from build123d import *

# Parameters (mm, degrees)
BOSS_EXTRUDE7_DEPTH = 3.6
SKETCH3_R           = 11.2
SKETCH3_R_2         = 5.25
BOSS_EXTRUDE8_DEPTH = 2
SKETCH4_R           = 2
CUT_EXTRUDE1_DEPTH  = 31.753353097
FILLET5_R           = 30
SKETCH5_R           = 1.8
BOSS_EXTRUDE9_DEPTH = 3.6
SKETCH6_R           = 2
CUT_EXTRUDE3_DEPTH  = 10


with BuildPart() as part:
    # Sketch1 → Boss-Extrude7 (new body)
    with BuildSketch(Plane(origin=(0, 0, 0), x_dir=(1, 0, 0), z_dir=(0, 1, 0))):
        with BuildLine():
            ThreePointArc((4.41085686, -11.428335039), (-4.687872046, -11.317524273), (-11.2, -4.962106408))
            Line((-11.2, -4.962106408), (-11.2, -17.382337649))
            ThreePointArc((-11.2, -17.382337649), (-8.730733729, -21.077855779), (-4.371572875, -20.210764774))
            Line((-4.371572875, -20.210764774), (4.41085686, -11.428335039))
        make_face()
        with BuildLine():
            ThreePointArc((7.91959592, -7.919595979), (-4.286054462, -10.347450756), (-11.2, 0))
            Line((-11.2, 0), (-11.2, -4.962106408))
            ThreePointArc((-11.2, -4.962106408), (-4.687872046, -11.317524273), (4.41085686, -11.428335039))
            Line((4.41085686, -11.428335039), (7.91959592, -7.919595979))
        make_face()
        with BuildLine():
            Line((11.428335039, -4.41085686), (7.91959592, -7.919595979))
            Line((7.91959592, -7.919595979), (4.41085686, -11.428335039))
            ThreePointArc((4.41085686, -11.428335039), (8.66205807, -8.66205807), (11.428335039, -4.41085686))
        make_face()
        with BuildLine():
            Line((4.962106408, 11.2), (0, 11.2))
            ThreePointArc((0, 11.2), (7.919595949, 7.919595949), (11.2, 0))
            ThreePointArc((11.2, 0), (10.347450756, -4.286054462), (7.91959592, -7.919595979))
            Line((7.91959592, -7.919595979), (11.428335039, -4.41085686))
            ThreePointArc((11.428335039, -4.41085686), (12.042831981, -2.243367532), (12.25, 0))
            ThreePointArc((12.25, 0), (10.267626393, 6.681193625), (4.962106408, 11.2))
        make_face()
        with BuildLine():
            Line((17.382337649, 11.2), (4.962106408, 11.2))
            ThreePointArc((4.962106408, 11.2), (10.267626393, 6.681193625), (12.25, 0))
            ThreePointArc((12.25, 0), (12.042831981, -2.243367532), (11.428335039, -4.41085686))
            Line((11.428335039, -4.41085686), (20.210764774, 4.371572875))
            ThreePointArc((20.210764774, 4.371572875), (21.077855779, 8.730733729), (17.382337649, 11.2))
        make_face()
        with BuildLine():
            ThreePointArc((-11.2, 0), (-7.919595949, 7.919595949), (0, 11.2))
            Line((0, 11.2), (4.962106408, 11.2))
            ThreePointArc((4.962106408, 11.2), (-8.66205807, 8.66205807), (-11.2, -4.962106408))
            Line((-11.2, -4.962106408), (-11.2, 0))
        make_face()
    extrude(amount=BOSS_EXTRUDE7_DEPTH)

    # Sketch3 → Boss-Extrude8 (add)
    # profile 1 of 2: a face of its own
    with BuildSketch(Plane(origin=(0, 3.6, 0), x_dir=(1, 0, 0), z_dir=(0, 1, 0))):
        with BuildLine():
            Line((-4.371572875, -20.210764774), (4.41085686, -11.428335039))
            ThreePointArc((4.41085686, -11.428335039), (8.66205807, -8.66205807), (11.428335039, -4.41085686))
            Line((11.428335039, -4.41085686), (20.210764774, 4.371572875))
            ThreePointArc((20.210764774, 4.371572875), (21.077855779, 8.730733729), (17.382337649, 11.2))
            Line((17.382337649, 11.2), (4.962106408, 11.2))
            ThreePointArc((4.962106408, 11.2), (-8.66205807, 8.66205807), (-11.2, -4.962106408))
            Line((-11.2, -4.962106408), (-11.2, -17.382337649))
            ThreePointArc((-11.2, -17.382337649), (-8.730733729, -21.077855779), (-4.371572875, -20.210764774))
        make_face()
        with Locations(Location((0, 0, 0), (0, 0, 270))):
            Circle(SKETCH3_R, mode=Mode.SUBTRACT)
    # profile 2 of 2: a face of its own
    with BuildSketch(Plane(origin=(0, 3.6, 0), x_dir=(1, 0, 0), z_dir=(0, 1, 0))):
        with Locations(Location((0, 0, 0), (0, 0, 270))):
            Circle(SKETCH3_R)
        with Locations(Location((0, 0, 0), (0, 0, 270))):
            Circle(SKETCH3_R_2, mode=Mode.SUBTRACT)
    extrude(amount=BOSS_EXTRUDE8_DEPTH)

    # Sketch4 → Cut-Extrude1 (cut, through all)
    with BuildSketch(Plane(origin=(0, 0, 0), x_dir=(1, 0, 0), z_dir=(0, 1, 0))):
        with Locations(Location((-7.2, -17.382337649, 0), (0, 0, 270))):
            Circle(SKETCH4_R)
        with Locations(Location((17.382337649, 7.2, 0), (0, 0, 270))):
            Circle(SKETCH4_R)
    extrude(amount=CUT_EXTRUDE1_DEPTH, mode=Mode.SUBTRACT)

    # Fillet5
    fillet5_edges = [part.edges().sort_by_distance(p)[0] for p in [
        (4.41085686, 2.8, 11.428335039),
        (-11.2, 2.8, 4.962106408),
        (4.962106408, 2.8, -11.2),
        (11.428335039, 2.8, 4.41085686),
    ]]
    fillet(fillet5_edges, radius=FILLET5_R)

    # Sketch5 → Boss-Extrude9 (add)
    with BuildSketch(Plane.XZ.offset(-3.6)):
        with Locations(Location((-8.1, 0, 0), (0, 0, 90))):
            Circle(SKETCH5_R)
        with Locations(Location((8.1, 0, 0), (0, 0, 90))):
            Circle(SKETCH5_R)
        with Locations(Location((0, -8.1, 0), (0, 0, 90))):
            Circle(SKETCH5_R)
        with Locations(Location((0, 8.1, 0), (0, 0, 90))):
            Circle(SKETCH5_R)
    extrude(amount=BOSS_EXTRUDE9_DEPTH)

    # Sketch6 → Cut-Extrude3 (cut)
    with BuildSketch(Plane.XZ):
        with Locations(Location((0, 8.1, 0), (0, 0, 90))):
            Circle(SKETCH6_R)
    cut_extrude3 = extrude(amount=-CUT_EXTRUDE3_DEPTH, mode=Mode.SUBTRACT)

    # Mirror1: Cut-Extrude3 across plane
    add(cut_extrude3.mirror(Plane(origin=(0, 0, 0), x_dir=(0.707106781186546, 0, 0.707106781186549), z_dir=(-0.707106781186549, 0, 0.707106781186546))), mode=Mode.SUBTRACT)


solid = part.part
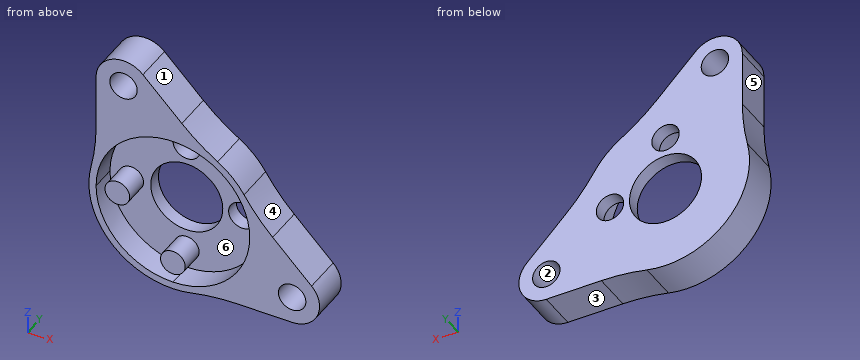
Model file for the job. Use its own axes, mm. Face numbers are marked on the shaded views. A direction names the side the tool comes from. Give positions to 0.01 mm unless a question says otherwise; leave off trailing zeros. Loops run counter-clockwise (first coordinate to the right, second up) from the corner with the lowest first, then second, coordinate; pieces in that order, holes last. Notation, with made-up numbers: (-32.75, 65) -> (-6.75, 65) arc R21 cw to (-6.75, 92) -> close; hole circle Ø3 at (19, 83.5). An arc over 180 degrees is marked (long way). Use a Markdown table: item, result. Add a question column.
(1) Slice it at C-C on z = -8.1. List the corners of the cut face in (x, y), and give its area (3 significant figures).
(2) Slice it at D-D on y = 5.2. List the corners of the cut face in (x, z), and give its area (3 significant figures).
(3) Slice it at B-B on x = -8.1. List the corners of the cut face in (y, z).
(4) Mould opens along Z. For the marked faces 1, 2 and 3 say: +Z half, -Z half, draft (parallel to the pull), parting line (faces both ways), or undercut.
(5) Tool access for the marked faces 4, 5 and 6: list every direction of +Z, -Z, +X, -X, +Y, -Y with a clear straight run to the whole face (end or side of a thin tool).
(6) Wall check: line 1 along Z through (x, y) = (-7.2, 3.25); line 2 along X through (y, z) = (2.2, 0.5); line 3 along X through (y, z) = (1, -1.5). Give the ranges that are in metal, low to high.
(7) Drop flat-ended pins along their axis: pin 1 Ø4.5 at (x, z) = (0, 8.1) entering from -Y; pin 2 Ø3.5 at (x, z) = (17.38, -7.2) entering from +Y; pin 3 Ø3 at (x, y) = (16.5, 4) entering from +Z; pin 4 Ø3 at (x, y) = (12, 3.5) entering from -Z. Give the stop position or say it passes through.
(8) Slice it at A-A on y = 1.5. List the corners of the cut face in (x, z), and give its area (3 significant figures).
Filled sheet:
| question | item | result |
|---|---|---|
| 1 | outline | (-9.19, 0) -> (-7.73, 0) -> (-7.73, 3.6) -> (-1.8, 3.6) -> (-1.8, 0) -> (1.8, 0) -> (1.8, 3.6) -> (7.73, 3.6) -> (7.73, 0) -> (15.6, 0) -> (15.6, 5.6) -> (-9.19, 5.6) -> close; (19.17, 0) -> (21.28, 0) -> (21.28, 5.6) -> (19.17, 5.6) -> close |
| 1 | area | 108 mm2 |
| 2 | outline | (-11.95, 2.71) arc R12.25 ccw to (2.71, -11.95) arc R30 cw to (9.36, -11.2) -> (17.38, -11.2) arc R4 ccw to (20.21, -4.37) -> (14.54, 1.3) arc R30 cw to (10.37, 6.53) arc R12.25 ccw to (6.53, 10.37) arc R30 cw to (1.3, 14.54) -> (-4.37, 20.21) arc R4 ccw to (-11.2, 17.38) -> (-11.2, 9.36) arc R30 cw to start; hole circle Ø4 at (-7.2, 17.38); hole circle Ø10.5 at (0, 0); hole circle Ø4 at (0, 8.1); hole circle Ø4 at (8.1, 0); hole circle Ø4 at (17.38, -7.2) |
| 2 | area | 564 mm2 |
| 3 | outline | (0, -9.19) -> (5.6, -9.19) -> (5.6, 15.6) -> (0, 15.6) -> (0, 7.73) -> (3.6, 7.73) -> (3.6, 1.8) -> (0, 1.8) -> (0, -1.8) -> (3.6, -1.8) -> (3.6, -7.73) -> (0, -7.73) -> close; (0, 19.17) -> (5.6, 19.17) -> (5.6, 21.28) -> (0, 21.28) -> close |
| 4 | face 1 | +Z half |
| 4 | face 2 | undercut |
| 4 | face 3 | -Z half |
| 5 | face 4 | +Z, +X, +Y, -Y |
| 5 | face 5 | +Z, -X, +Y, -Y |
| 5 | face 6 | -Y |
| 6 | line 1 | -9.91 to -8.58, -1.56 to 1.56, 8.58 to 15.38, 19.38 to 21.38 |
| 6 | line 2 | -12.24 to -11.19, -9.83 to -6.37, 11.19 to 15.34 |
| 6 | line 3 | -12.16 to -11.1, -9.09 to -7.11, 11.1 to 17.34 |
| 7 | pin 1 | y = 3.6 |
| 7 | pin 2 | through |
| 7 | pin 3 | z = 0.84 |
| 7 | pin 4 | z = -11.2 |
| 8 | outline | (-11.95, 2.71) arc R12.25 ccw to (2.71, -11.95) arc R30 cw to (9.36, -11.2) -> (17.38, -11.2) arc R4 ccw to (20.21, -4.37) -> (14.54, 1.3) arc R30 cw to (10.37, 6.53) arc R12.25 ccw to (6.53, 10.37) arc R30 cw to (1.3, 14.54) -> (-4.37, 20.21) arc R4 ccw to (-11.2, 17.38) -> (-11.2, 9.36) arc R30 cw to start; circle Ø3.6 at (-8.1, 0); circle Ø3.6 at (0, -8.1); hole circle Ø22.4 at (0, 0); hole circle Ø4 at (-7.2, 17.38); hole circle Ø4 at (17.38, -7.2) |
| 8 | area | 302 mm2 |
